from build123d import *

# Parameters (mm, degrees)
ESBO_O1_W                      = 100
ESBO_O1_H                      = 120
RESSALTO_EXTRUS_O1_DEPTH       = 3
ARESTA_FLANGE1_STRIP_W         = 13.8
ARESTA_FLANGE1_STRIP_H         = 3
ARESTA_FLANGE1_STRIP_CUT_DEPTH = 100
ARESTA_FLANGE1_DEPTH           = 100
ARESTA_FLANGE2_STRIP_W         = 13.8
ARESTA_FLANGE2_STRIP_H         = 3
ARESTA_FLANGE2_STRIP_CUT_DEPTH = 100
ARESTA_FLANGE2_DEPTH           = 100
CORTE_EXTRUS_O1_DEPTH          = 171.002941151
ESBO_O13_R                     = 10
CORTE_EXTRUS_O2_DEPTH          = 171.002941151
DESDOBRAR1_START               = 3
DESDOBRAR1_OUTLINE_W           = 100
DESDOBRAR1_OUTLINE_H           = 126
DESDOBRAR1_DEPTH               = 53
DESDOBRAR1_2_OUTLINE_R         = 10
DESDOBRAR1_2_DEPTH             = 3
DOBRAR1_START                  = -175
DOBRAR1_OUTLINE_W              = 100
DOBRAR1_OUTLINE_H              = 3
DOBRAR1_DEPTH                  = 52
DOBRAR1_START_2                = 3
DOBRAR1_2_OUTLINE_W            = 100
DOBRAR1_2_OUTLINE_H            = 3
DOBRAR1_2_DEPTH                = 52
DOBRAR1_START_3                = -123
DOBRAR1_3_OUTLINE_R            = 10
DOBRAR1_3_DEPTH                = 3.9
DOBRAR1_START_4                = -0.9
DOBRAR1_4_OUTLINE_R            = 10
DOBRAR1_4_DEPTH                = 3.9
DOBRAR1_START_5                = -1
DOBRAR1_5_DEPTH                = 102


with BuildPart() as part:
    # Esboço1 → Ressalto-extrusão1 (new body)
    with BuildSketch(Plane(origin=(0, 0, 0), x_dir=(1, 0, 0), z_dir=(0, 1, 0))):
        with Locations((50, 60)):
            Rectangle(ESBO_O1_W, ESBO_O1_H)
    extrude(amount=RESSALTO_EXTRUS_O1_DEPTH)

    # Aresta-Flange1: sheet metal written as solids
    # Aresta-Flange1 strip (on a plane across the edge) → Aresta-Flange1 strip cut (cut)
    with BuildSketch(Plane(origin=(0, 3, 0), x_dir=(0, 0, -1), z_dir=(1, 0, 0))):
        with Locations((-6, -1.5)):
            Rectangle(ARESTA_FLANGE1_STRIP_W, ARESTA_FLANGE1_STRIP_H)
    extrude(amount=ARESTA_FLANGE1_STRIP_CUT_DEPTH, mode=Mode.SUBTRACT)

    # Aresta-Flange1 section (on a plane across the edge) → Aresta-Flange1 (add)
    with BuildSketch(Plane(origin=(0, 3, 0), x_dir=(0, 0, -1), z_dir=(1, 0, 0))):
        with BuildLine():
            Line((-3, 0.9), (-3, 52))
            Line((-3, 52), (0, 52))
            Line((0, 52), (0, 0.9))
            ThreePointArc((0, 0.9), (0.263603897, 0.263603897), (0.9, 0))
            Line((0.9, 0), (0.9, -3))
            ThreePointArc((0.9, -3), (-1.857716447, -1.857716447), (-3, 0.9))
        make_face()
    extrude(amount=ARESTA_FLANGE1_DEPTH)

    # Aresta-Flange2: sheet metal written as solids
    # Aresta-Flange2 strip (on a plane across the edge) → Aresta-Flange2 strip cut (cut)
    with BuildSketch(Plane(origin=(100, 3, -120), x_dir=(0, 0, 1), z_dir=(-1, 0, 0))):
        with Locations((-6, -1.5)):
            Rectangle(ARESTA_FLANGE2_STRIP_W, ARESTA_FLANGE2_STRIP_H)
    extrude(amount=ARESTA_FLANGE2_STRIP_CUT_DEPTH, mode=Mode.SUBTRACT)

    # Aresta-Flange2 section (on a plane across the edge) → Aresta-Flange2 (add)
    with BuildSketch(Plane(origin=(100, 3, -120), x_dir=(0, 0, 1), z_dir=(-1, 0, 0))):
        with BuildLine():
            Line((-3, 0.9), (-3, 52))
            Line((-3, 52), (0, 52))
            Line((0, 52), (0, 0.9))
            ThreePointArc((0, 0.9), (0.263603897, 0.263603897), (0.9, 0))
            Line((0.9, 0), (0.9, -3))
            ThreePointArc((0.9, -3), (-1.857716447, -1.857716447), (-3, 0.9))
        make_face()
    extrude(amount=ARESTA_FLANGE2_DEPTH)

    # Esboço11 → Corte-extrusão1 (cut, through all)
    with BuildSketch(Plane.XY.offset(3)):
        with BuildLine():
            Line((0, 55), (0, 8))
            Line((0, 8), (38.984187706, 50.180956709))
            ThreePointArc((38.984187706, 50.180956709), (43.988109725, 53.74253162), (50, 55))
            Line((50, 55), (0, 55))
        make_face()
        with BuildLine():
            Line((61.015812294, 50.180956709), (100, 8))
            Line((100, 8), (100, 55))
            Line((100, 55), (50, 55))
            ThreePointArc((50, 55), (56.011890275, 53.74253162), (61.015812294, 50.180956709))
        make_face()
    extrude(amount=-CORTE_EXTRUS_O1_DEPTH, mode=Mode.SUBTRACT)

    # Esboço13 → Corte-extrusão2 (cut, through all)
    with BuildSketch(Plane.XY.offset(3)):
        with Locations((50, 40)):
            Circle(ESBO_O13_R)
    extrude(amount=-CORTE_EXTRUS_O2_DEPTH, mode=Mode.SUBTRACT)

    # Desdobrar1: read off the stored shape, not the designer's step
    # Desdobrar1 outline → Desdobrar1 (cut)
    with BuildSketch(Plane(origin=(0, 0, 0), x_dir=(1, 0, 0), z_dir=(0, 1, 0)).offset(DESDOBRAR1_START)):
        with Locations((50, 60)):
            Rectangle(DESDOBRAR1_OUTLINE_W, DESDOBRAR1_OUTLINE_H)
    extrude(amount=DESDOBRAR1_DEPTH, mode=Mode.SUBTRACT)

    # Desdobrar1 2 outline → Desdobrar1 2 (add)
    with BuildSketch(Plane(origin=(0, 0, 0), x_dir=(1, 0, 0), z_dir=(0, 1, 0))):
        with BuildLine():
            Line((0, -6.969911184), (38.984187706, -49.150867893))
            ThreePointArc((38.984187706, -49.150867893), (50, -53.969911184), (61.015812294, -49.150867893))
            Line((61.015812294, -49.150867893), (100, -6.969911184))
            Line((100, -6.969911184), (100, 126.969911184))
            Line((100, 126.969911184), (61.015812294, 169.150867893))
            ThreePointArc((61.015812294, 169.150867893), (50, 173.969911184), (38.984187706, 169.150867893))
            Line((38.984187706, 169.150867893), (0, 126.969911184))
            Line((0, 126.969911184), (0, -6.969911184))
        make_face()
        with Locations((50, 158.969911184)):
            Circle(DESDOBRAR1_2_OUTLINE_R, mode=Mode.SUBTRACT)
        with Locations((50, -38.969911184)):
            Circle(DESDOBRAR1_2_OUTLINE_R, mode=Mode.SUBTRACT)
    extrude(amount=DESDOBRAR1_2_DEPTH)

    # Dobrar1: read off the stored shape, not the designer's step
    # Dobrar1 outline → Dobrar1 (cut)
    with BuildSketch(Plane.XY.offset(DOBRAR1_START)):
        with Locations((50, 1.5)):
            Rectangle(DOBRAR1_OUTLINE_W, DOBRAR1_OUTLINE_H)
    extrude(amount=DOBRAR1_DEPTH, mode=Mode.SUBTRACT)

    # Dobrar1 2 outline → Dobrar1 2 (cut)
    with BuildSketch(Plane.XY.offset(DOBRAR1_START_2)):
        with Locations((50, 1.5)):
            Rectangle(DOBRAR1_2_OUTLINE_W, DOBRAR1_2_OUTLINE_H)
    extrude(amount=DOBRAR1_2_DEPTH, mode=Mode.SUBTRACT)

    # Dobrar1 3 outline → Dobrar1 3 (add)
    with BuildSketch(Plane.XY.offset(DOBRAR1_START_3)):
        with BuildLine():
            Line((0, 8), (0, 3))
            Line((0, 3), (100, 3))
            Line((100, 3), (100, 8))
            Line((100, 8), (61.015812294, 50.180956709))
            ThreePointArc((61.015812294, 50.180956709), (50, 55), (38.984187706, 50.180956709))
            Line((38.984187706, 50.180956709), (0, 8))
        make_face()
        with Locations((50, 40)):
            Circle(DOBRAR1_3_OUTLINE_R, mode=Mode.SUBTRACT)
    extrude(amount=DOBRAR1_3_DEPTH)

    # Dobrar1 4 outline → Dobrar1 4 (add)
    with BuildSketch(Plane.XY.offset(DOBRAR1_START_4)):
        with BuildLine():
            Line((0, 8), (0, 3))
            Line((0, 3), (100, 3))
            Line((100, 3), (100, 8))
            Line((100, 8), (61.015812294, 50.180956709))
            ThreePointArc((61.015812294, 50.180956709), (50, 55), (38.984187706, 50.180956709))
            Line((38.984187706, 50.180956709), (0, 8))
        make_face()
        with Locations((50, 40)):
            Circle(DOBRAR1_4_OUTLINE_R, mode=Mode.SUBTRACT)
    extrude(amount=DOBRAR1_4_DEPTH)

    # Dobrar1 5 outline → Dobrar1 5 (cut)
    with BuildSketch(Plane.YZ.offset(DOBRAR1_START_5)):
        with BuildLine():
            Line((56, 0), (3.9, 0))
            ThreePointArc((3.9, 0), (3.263603897, -0.263603897), (3, -0.9))
            Line((3, -0.9), (56, -0.9))
            Line((56, -0.9), (56, 0))
        make_face()
        with BuildLine():
            Line((3.9, 3), (56, 2.999999983))
            Line((56, 2.999999983), (56, 5))
            Line((56, 5), (4e-08, 5))
            Line((4e-08, 5), (0, -0.9))
            ThreePointArc((0, -0.9), (1.142283553, 1.857716447), (3.9, 3))
        make_face()
        with BuildLine():
            Line((56, -120), (56, -119.1))
            Line((56, -119.1), (3, -119.1))
            ThreePointArc((3, -119.1), (3.263603897, -119.736396103), (3.9, -120))
            Line((3.9, -120), (56, -120))
        make_face()
        with BuildLine():
            Line((56, -124), (56, -122.999999983))
            Line((56, -122.999999983), (3.9, -123))
            ThreePointArc((3.9, -123), (1.142283553, -121.857716447), (0, -119.1))
            Line((0, -119.1), (4e-08, -124))
            Line((4e-08, -124), (56, -124))
        make_face()
    extrude(amount=DOBRAR1_5_DEPTH, mode=Mode.SUBTRACT)


solid = part.part
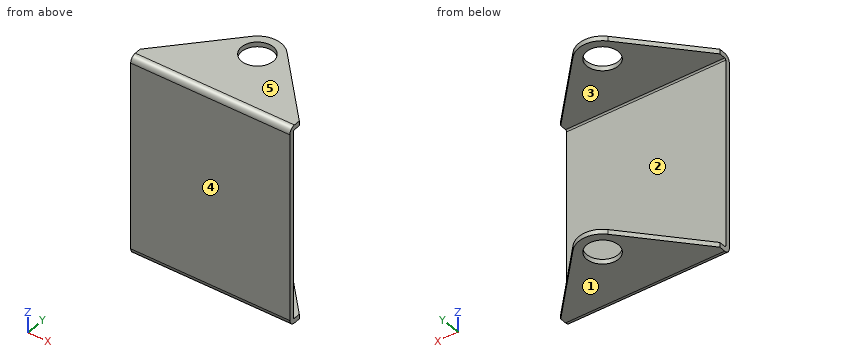
Design review of the part built by this model. Coordinates are the model's own, in mm. Face numbers are marked on the shaded views. A direction names the side the tool comes from. Round coordinates to 2 decimals unless told otherwise and drop trailing zeros. Write each loop counter-clockwise with the first axis right and the second up, starting at its lowest first coordinate (ties: lowest second). Pieces come first, ordered by that corner, then holes.
Item 1: For pin 1 Ø12 at (x, y) = (50, 40) entering from -Z; pin 2 Ø2 at (x, z) = (65.5, -70.5) entering from +Y, all flat-tipped, find the tip position at first contact; note any pin that passes through.
Item 2: Consider section C-C on y = 40. Give the boundary of the cut face in (x, z), and give its area (3 significant figures).
Item 3: Consider section B-B on x = 50. Give the boundary of the cut face in (y, z), and give its area (3 significant figures).
Item 4: Consider section A-A on y = 6. Give the boundary of the cut face in (x, z).
Item 5: For the marked faces 1 and 2, list the 3-axis set-ups (+Z, -Z, +X, -X, +Y, -Y) from which the entire face can be reached by the end or side of a thin tool; tool diameter is ignored.
Item 6: Draft analysis for pull direction Z (two halves, no side actions). For the marked faces 3, 4 and 5, state which applies: released by +Z, released by -Z, zero draft, split by the parting line, or undercut.
Item 7: Consider section D-D on x = 27.5. Give the boundary of the cut face in (y, z), and give its area (3 significant figures).
Item 8: Wall thickness on L1, parallel to Z at x = 11, y = 10; L2, parallel to Y at x = 50, z = 1.55; L3, parallel to Y at x = 50, z = 1: over which ranges is each line inside the solid? List them lowest first.
Check values:
1. pin 1: passes through
1. pin 2: stops at y = 3
2. outline: (29.57, -123) - (40, -123) - (40, -120) - (29.57, -120) - close; (29.57, 0) - (40, 0) - (40, 3) - (29.57, 3) - close; (60, -123) - (70.43, -123) - (70.43, -120) - (60, -120) - close; (60, 0) - (70.43, 0) - (70.43, 3) - (60, 3) - close
2. area: 125 mm2
3. outline: (0, -119.1) arc R3.9 ccw to (3.9, -123) - (30, -123) - (30, -120) - (3.9, -120) arc R0.9 cw to (3, -119.1) - (3, -0.9) arc R0.9 cw to (3.9, 0) - (30, 0) - (30, 3) - (3.9, 3) arc R3.9 ccw to (0, -0.9) - close; (50, -123) - (55, -123) - (55, -120) - (50, -120) - close; (50, 0) - (55, 0) - (55, 3) - (50, 3) - close
3. area: 564 mm2
4. outline: (0, -123) - (100, -123) - (100, -120) - (0, -120) - close; (0, 0) - (100, 0) - (100, 3) - (0, 3) - close
5. face 1: -Z, +X, -X, +Y, -Y
5. face 2: +X, -X, +Y
6. face 3: undercut
6. face 4: zero draft
6. face 5: released by +Z
7. outline: (0, -119.1) arc R3.9 ccw to (3.9, -123) - (37.76, -123) - (37.76, -120) - (3.9, -120) arc R0.9 cw to (3, -119.1) - (3, -0.9) arc R0.9 cw to (3.9, 0) - (37.76, 0) - (37.76, 3) - (3.9, 3) arc R3.9 ccw to (0, -0.9) - close
7. area: 580 mm2
8. L1: z = -123 to -120, 0 to 3
8. L2: y = 0.87 to 30, 50 to 55
8. L3: y = 0.49 to 30, 50 to 55
